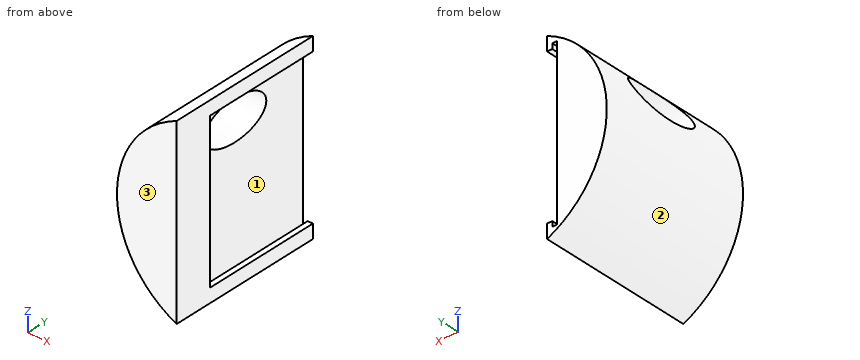
from build123d import *

# Parameters (mm, degrees)
BOSS_EXTRUDE1_DEPTH     = 39
CUT_EXTRUDE1_DEPTH      = 29.4
SKETCH3_RX              = 9
SKETCH3_RY              = 5
CUT_EXTRUDE2_DEPTH      = 3.5
CUT_EXTRUDE2_DEPTH_BACK = 13.5


with BuildPart() as part:
    # Sketch1 → Boss-Extrude1 (new body)
    with BuildSketch(Plane(origin=(0, 0, 0), x_dir=(1, 0, 0), z_dir=(0, 1, 0))):
        with BuildLine():
            Line((-10, 22.912878475), (-10, -22.912878475))
            ThreePointArc((-10, -22.912878475), (-25, 0), (-10, 22.912878475))
        make_face()
    extrude(amount=BOSS_EXTRUDE1_DEPTH)

    # Sketch2 → Cut-Extrude1 (cut)
    with BuildSketch(Plane(origin=(0, 39, 0), x_dir=(1, 0, 0), z_dir=(0, 1, 0))):
        Polygon((-10, 19.412878475), (-11.3, 19.412878475), (-11.3, 20.712878475), (-12.5, 20.712878475), (-12.5, -20.712878475), (-11.3, -20.712878475), (-11.3, -19.412878475), (-10, -19.412878475), align=None)
    extrude(amount=-CUT_EXTRUDE1_DEPTH, mode=Mode.SUBTRACT)

    # Sketch3 → Cut-Extrude2 (cut, two sides)
    with BuildSketch(Plane(origin=(-12.5, 0, 0), x_dir=(0, 0, -1), z_dir=(1, 0, 0))) as cut_extrude2_sk:
        with Locations(Location((-12.420207371, 19.5), (0, 0, 90))):
            Ellipse(SKETCH3_RX, SKETCH3_RY)
    extrude(amount=CUT_EXTRUDE2_DEPTH, mode=Mode.SUBTRACT)
    extrude(cut_extrude2_sk.sketch, amount=-CUT_EXTRUDE2_DEPTH_BACK, mode=Mode.SUBTRACT)


solid = part.part
Here's how the part is built. I have some questions about the finished solid (model axes, mm). Face numbers are marked on the shaded views. Round coordinates to 2 decimals unless told otherwise and drop trailing zeros. Order: outer loops, then holes, each group sorted by start corner. A loop starts at its lowest first (then second) coordinate and runs counter-clockwise, first axis right, second up. Notation, with made-up numbers: (-11, -25) -> (28, -25) arc R25 ccw to (28, -7) -> close; hole circle Ø11 at (77.5, 44.25). An arc over 180 degrees is marked (long way). Return JSON: item names as keys, results as strings.
Q1. If we mould it in two halves opening along Z, with no side actions, what happens to the marked faces 1, 2 and 3? For each: released by +Z, released by -Z, zero draft, split by the parting line, or undercut.
Filled sheet:
{"face 1": "undercut", "face 2": "split by the parting line", "face 3": "zero draft"}
Q2. If we section it at B-B on y = 34: List the corners of the cut face in (x, z) for me.
Filled sheet:
{"outline": "(-12.5, -20.71) -> (-12.5, 20.71) -> (-11.3, 20.71) -> (-11.3, 19.41) -> (-10, 19.41) -> (-10, 22.91) arc R25 ccw to (-10, -22.91) -> (-10, -19.41) -> (-11.3, -19.41) -> (-11.3, -20.71) -> close"}
Q3. I need wall thicknesses on line 1 along Y through (x, z) = (-12.25, 2); line 2 along Z through (x, y) = (-11.75, 10); line 3 along X through (y, z) = (12.5, 20). Which ranges of each line are inside material? Lowest first, please. Write a range as from..to.
Filled sheet:
{"line 1": "y = 0..9.6", "line 2": "z = -22.07..-20.71, 20.71..22.07", "line 3": "x = -15..-12.5, -11.3..-10"}
Q4. If we section it at C-C on y = 7: List the corners of the cut face in (x, z) for me.
Filled sheet:
{"outline": "(-10, -22.91) -> (-10, 22.91) arc R25 ccw to start"}
Q5. If we section it at D-D on z = -8.5: List the corners of the cut face in (x, y) for me.
Filled sheet:
{"outline": "(-23.51, 0) -> (-10, 0) -> (-10, 9.6) -> (-12.5, 9.6) -> (-12.5, 39) -> (-23.51, 39) -> close"}
Q6. For pin 1 Ø2 at (y, z) = (33.5, 8) entering from +X; pin 2 Ø1 at (x, y) = (-14.5, 9.5) entering from -Z; pin 3 Ø1.4 at (y, z) = (28.5, -20.5) entering from -X, each with a flat end and sliding along its axis, tell me the tip position at first contact or that it passes through.
Filled sheet:
{"pin 1": "stops at x = -12.5", "pin 2": "stops at z = -20.71", "pin 3": "stops at x = -15.26"}
Q7. If we section it at A-A on z = 0: List the corners of the cut face in (x, y) for me.
Filled sheet:
{"outline": "(-25, 0) -> (-10, 0) -> (-10, 9.6) -> (-12.5, 9.6) -> (-12.5, 39) -> (-25, 39) -> close"}
